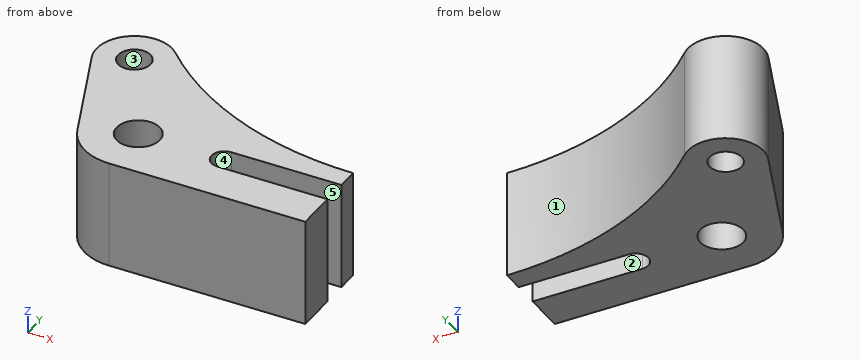
from build123d import *

# Parameters (mm, degrees)
SKETCH1_R           = 7.5
SKETCH1_R_2         = 10
BOSS_EXTRUDE1_DEPTH = 25


with BuildPart() as part:
    # Sketch1 → Boss-Extrude1 (new, symmetric)
    with BuildSketch(Plane.XY):
        with BuildLine():
            ThreePointArc((40, 6), (34, 0), (40, -6))
            Line((40, -6), (91.012125426, -6))
            Line((91.012125426, -6), (91.012125426, -25))
            Line((91.012125426, -25), (0, -25))
            ThreePointArc((0, -25), (-13.950413836, -20.745745439), (-23.152938737, -9.430876304))
            Line((-23.152938737, -9.430876304), (-43.707057116, 41.029783795))
            ThreePointArc((-43.707057116, 41.029783795), (-37.175167009, 62.213617319), (-15.118136149, 59.998266157))
            ThreePointArc((-15.118136149, 59.998266157), (33.56763081, 27.43546616), (91.012125426, 16))
            Line((91.012125426, 16), (91.012125426, 6))
            Line((91.012125426, 6), (40, 6))
        make_face()
        with Locations((-27.5, 47.631397208)):
            Circle(SKETCH1_R, mode=Mode.SUBTRACT)
        Circle(SKETCH1_R_2, mode=Mode.SUBTRACT)
    extrude(amount=BOSS_EXTRUDE1_DEPTH, both=True)


solid = part.part
The listing builds one solid part. Answer for the finished solid, in the listing's coordinates (mm). Face numbers are marked on the shaded views. A direction names the side the tool comes from. Give positions to 0.01 mm unless a question says otherwise; leave off trailing zeros. Write each loop counter-clockwise with the first axis right and the second up, starting at its lowest first coordinate (ties: lowest second). Pieces come first, ordered by that corner, then holes.
1) Section D-D (y = 20) is taken. Write down the section's boundary in (x, z).
2) For a pull along X with two mould halves and no side action, classify the marked faces 3, 4 and 5 as pulls with the +X half, pulls with the -X half, needs draft (parallel to the pull), parting line crosses it, or undercut.
3) Given P1, Ø12, axis at x = 60, z = 7.5, coming from the +Y side; P2, Ø12, axis at x = 0, y = 0, coming from the +Z side; P3, Ø3, axis at y = 42, z = -9.5, coming from the -X side; P4, Ø2, axis at x = -13, z = -17.5, coming from the +Y side, each flat-ended and moving along its own axis, determine where each tip first touches the part or whether it passes through.
4) Find the intervals of material crossed by L1, parallel to Y at x = -27, z = 1; L2, parallel to Y at x = 38.5, z = 7.5; L3, parallel to X at y = 43, z = 1, in increasing order.
5) Section A-A (x = 76) is taken. Write down the section's boundary in (y, z).
6) Section C-C (z = 0.5) is taken. Write down the section's boundary in (x, y).
7) A tool of negligible diameter and unlimited length cuts with its end or side. For the marked faces 1 and 2, from which of +Z, -Z, +X, -X, +Y, -Y can it reach the whole face along a straight path? Write none if from no direction.
8) Section B-B (y = 0) is taken. Write down the section's boundary in (x, z), and give its area (3 significant figures).
Response:
1. outline: (-35.14, -25) - (56.6, -25) - (56.6, 25) - (-35.14, 25) - close
2. face 3: undercut
2. face 4: pulls with the +X half
2. face 5: needs draft
3. P1: stops at y = 20.64
3. P2: passes through
3. P3: stops at x = -44.51
3. P4: stops at y = 58.89
4. L1: y = 0.01 to 40.15, 55.11 to 65.12
4. L2: y = -25 to -5.81, 5.81 to 25.49
4. L3: x = -44.38 to -33.4, -21.6 to 5.16
5. outline: (-25, -25) - (-6, -25) - (-6, 25) - (-25, 25) - close; (6, -25) - (16.75, -25) - (16.75, 25) - (6, 25) - close
6. outline: (-43.71, 41.03) - (-23.15, -9.43) arc R25 ccw to (0, -25) - (91.01, -25) - (91.01, -6) - (40, -6) arc R6 cw to (40, 6) - (91.01, 6) - (91.01, 16) arc R150 cw to (-15.12, 60) arc R17.5 ccw to start; hole circle Ø15 at (-27.5, 47.63); hole circle Ø20 at (0, 0)
7. face 1: +Z, -Z, +X, +Y
7. face 2: +Z, -Z, +X
8. outline: (-26.99, -25) - (-10, -25) - (-10, 25) - (-26.99, 25) - close; (10, -25) - (34, -25) - (34, 25) - (10, 25) - close
8. area: 2,050 mm2
